Input: part model. Units: mm. Frame: model coordinates. Give positions to 0.01 mm unless a question says otherwise; leave off trailing zeros. Loops run counter-clockwise (first coordinate to the right, second up) from the corner with the lowest first, then second, coordinate; pieces in that order, holes last. Notation, with made-up numbers: M -38,71.5 L 18,71.5 A19 ccw 18,76.5 Z; hole C 39.5,31 d11. An arc over 180 degrees is marked long. Use a Markdown table: item, result. Add a question column.
Autodesk Inventor part; units mm, degrees
ref_plane "YZ Plane" through (0, 0, 0) normal (1, 0, 0) x (0, 1, 0)
ref_plane "XZ Plane" through (0, 0, 0) normal (0, 1, 0) x (-1, 0, 0)
ref_plane "XY Plane" through (0, 0, 0) normal (0, 0, 1) x (1, 0, 0)
sketch "Sketch4" plane through (0, 0, 0) normal (0, 0, 1) x (1, 0, 0)
  line L0 (0, 0) -> (-60, 0)
  line L1 (-60, 0) -> (-60, 20)
  line L2 (-60, 20) -> (0, 20)
  line L3 (0, 20) -> (0, 0)
  dimension "d37" = 60
  dimension "d38" = 20
extrude "Extrusion2" add sketch "Sketch4" along normal blind 10
hole "Hole2" at (-30, 10, 10) direction (0, 0, -1) diameter 10 depth 10 tip angle 118
hole "Hole3" at (-55, 15, 10) direction (0, 0, -1) diameter 4.134 depth 14.2 tip angle 118
hole "Hole4" at (-5, 15, 10) direction (0, 0, -1) diameter 4.134 depth 14.2 tip angle 118
hole "Hole5" at (-5, 5, 10) direction (0, 0, -1) diameter 4.343 depth 16.265 tip angle 118
hole "Hole6" at (-55, 5, 10) direction (0, 0, -1) diameter 4.134 depth 14.2 tip angle 118
properties part number "GARFO" material "Aluminium AW-7020"
1) Section query C-C, the plane z = 7. Return the cut outline in (x, y), and give its area (3 significant figures).
2) Section query D-D, the plane x = -55. Return the cut outline in (y, z).
3) Pull-direction query (X, two-part tool) for faces 1 (the flat face through (-37, 10, 0)), 2 (the flat face through (0, 10, 5)), 3 (the flat face through (-60, 10, 5)), 4 (the cylindrical face through (-57.05, 5.27, 4.93)); classes: pulls with the +X half, pulls with the -X half, needs draft (parallel to the pull), parting line crosses it, or undercut.
4) Ray query, line 1 (Y direction, x = -5, z = 4.25); line 2 (Y direction, x = -55, z = 4); line 3 (Y direction, x = -30, z = 4.25). Return the intervals inside material, ascending. Write a range as [from, to].
5) Section query A-A, the plane y = 10. Return the cut outline in (x, z), and give its area (3 significant figures).
6) Section query B-B, the plane x = -30. Return the cut outline in (y, z), and give its area (3 significant figures).
Entries:
| question | item | result |
|---|---|---|
| 1 | outline | M -60,0 L 0,0 L 0,20 L -60,20 Z; hole C -55,5 d4.13; hole C -55,15 d4.13; hole C -30,10 d10; hole C -5,5 d4.34; hole C -5,15 d4.13 |
| 1 | area | 1,070 mm² |
| 2 | outline | M 0,0 L 2.93,0 L 2.93,10 L 0,10 Z; M 7.07,0 L 12.93,0 L 12.93,10 L 7.07,10 Z; M 17.07,0 L 20,0 L 20,10 L 17.07,10 Z |
| 3 | face 1 | needs draft |
| 3 | face 2 | pulls with the +X half |
| 3 | face 3 | pulls with the -X half |
| 3 | face 4 | undercut |
| 4 | line 1 | y = [0, 2.83], [7.17, 12.93], [17.07, 20] |
| 4 | line 2 | y = [0, 2.93], [7.07, 12.93], [17.07, 20] |
| 4 | line 3 | y = [0, 5], [15, 20] |
| 5 | outline | M -60,0 L -35,0 L -35,10 L -60,10 Z; M -25,0 L 0,0 L 0,10 L -25,10 Z |
| 5 | area | 500 mm² |
| 6 | outline | M 0,0 L 5,0 L 5,10 L 0,10 Z; M 15,0 L 20,0 L 20,10 L 15,10 Z |
| 6 | area | 100 mm² |
